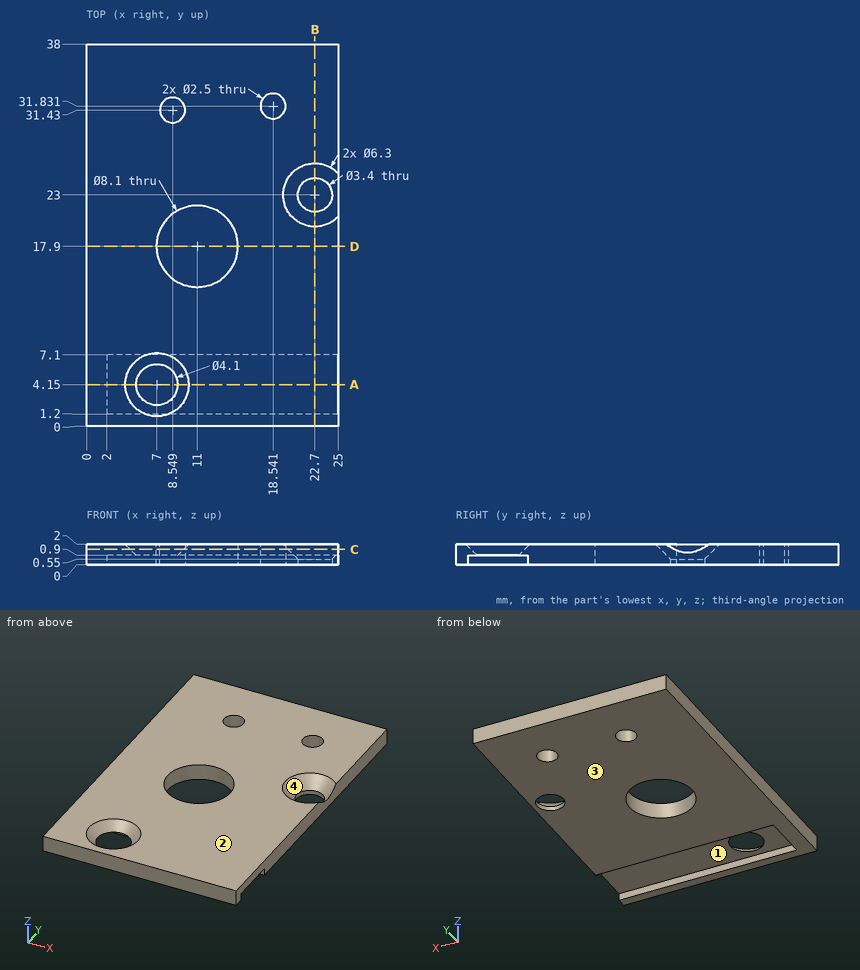
Job drawing, mm, ordinate dimensions from the low corner. One solid piece. A direction names the side the tool comes from. Round coordinates to 2 decimals unless told otherwise and drop trailing zeros. Order: outer loops, then holes, each group sorted by start corner. A loop starts at its lowest first (then second) coordinate and runs counter-clockwise, first axis right, second up. Notation, with made-up numbers: (-33.75, 74.25) - (-14.75, 74.25) arc R26 ccw to (-14.75, 105.25) - close; hole circle Ø8 at (20.25, 71.25). An arc over 180 degrees is marked (long way). Use CSV: the item, a comma, the result in double quotes. Start each with the question number.
1) Saw through at A-A (y = 4.15). List the corners of the cut face in (x, z).
2) Tool access for the marked faces 1 and 2: list every direction of +Z, -Z, +X, -X, +Y, -Y with a clear straight run to the whole face (end or side of a thin tool).
3) Two-plate mould, pull along Y, no slides. Class the marked faces 3 and 4: pulls with the +Y half, pulls with the -Y half, needs draft (parallel to the pull), parting line crosses it, or undercut.
4) Saw through at D-D (y = 17.9). List the corners of the cut face in (x, z), and give its area (3 significant figures).
5) Wall check: L1, parallel to Y at x = 22.7, z = 0.45; L2, parallel to Y at x = 11, z = 0.8; L3, parallel to X at y = 31, z = 0.7 (1 decimal). Give the ranges that are in metal, low to high. Write a range as [from, to].
6) Saw through at C-C (z = 1.5). List the corners of the cut face in (x, y), and give its area (3 significant figures).
7) Saw through at B-B (x = 22.7). List the corners of the cut face in (y, z).
8) Pin check, flat tips, straight feed: pin 1 Ø3 at (x, y) = (18.54, 31.83) entering from +Z; pin 2 Ø2 at (x, y) = (22.7, 23) entering from -Z. Stop position of each tip, or through.
Values follow:
1,outline,"(0, 0) - (2, 0) - (2, 0.9) - (4.95, 0.9) - (3.85, 2) - (0, 2) - close; (9.05, 0.9) - (25, 0.9) - (25, 2) - (10.15, 2) - close"
2,face 1,"-Z, +X"
2,face 2,"+Z, +X, -X, +Y, -Y"
3,face 3,"needs draft"
3,face 4,"undercut"
4,outline,"(0, 0) - (6.95, 0) - (6.95, 2) - (0, 2) - close; (15.05, 0) - (25, 0) - (25, 2) - (15.05, 2) - close"
4,area,"33.8 mm2"
5,L1,"y = [0, 1.2], [7.1, 21.3], [24.7, 38]"
5,L2,"y = [0, 1.2], [7.1, 13.85], [21.95, 38]"
5,L3,"x = [0, 7.4], [9.7, 17.6], [19.5, 25]"
6,outline,"(0, 0) - (25, 0) - (25, 21.68) arc R2.65 cw (long way) to (25, 24.32) - (25, 38) - (0, 38) - close; hole circle Ø5.3 at (7, 4.15); hole circle Ø8.1 at (11, 17.9); hole circle Ø2.5 at (8.55, 31.43); hole circle Ø2.5 at (18.54, 31.83)"
6,area,"845 mm2"
7,outline,"(0, 0) - (1.2, 0) - (1.2, 0.9) - (7.1, 0.9) - (7.1, 0) - (21.3, 0) - (21.3, 0.55) - (19.85, 2) - (0, 2) - close; (24.7, 0) - (38, 0) - (38, 2) - (26.15, 2) - (24.7, 0.55) - close"
8,pin 1,"stops at z = 2"
8,pin 2,"passes through"
